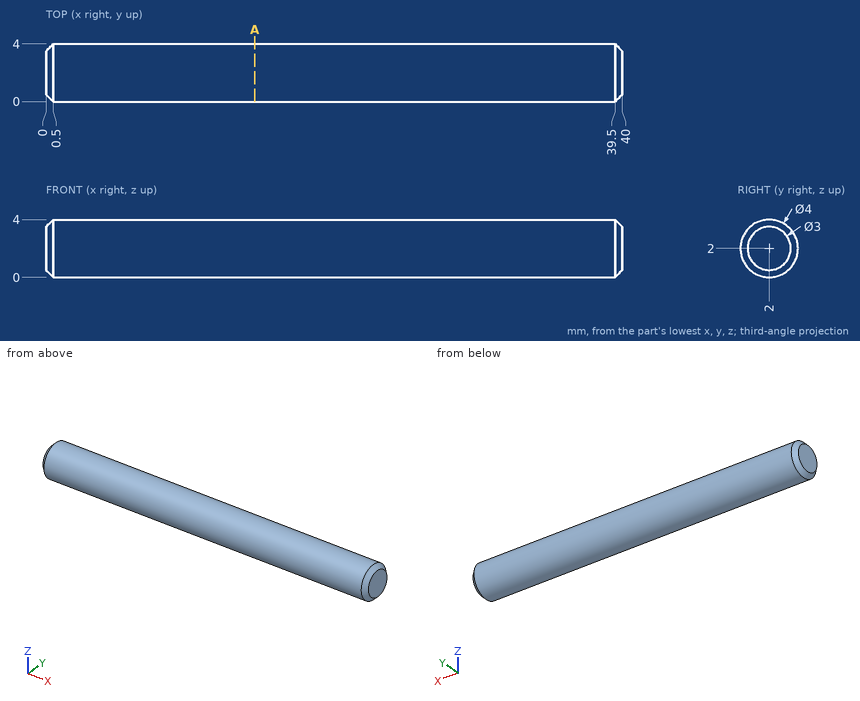
For this review, use the dimensioned drawing (mm, ordinates from the lowest corner) and the shaded views. Coordinates: 2 decimals unless noted, no trailing zeros. Write each loop counter-clockwise with the first axis right and the second up, starting at its lowest first coordinate (ties: lowest second). Pieces come first, ordered by that corner, then holes. Notation, with made-up numbers: (73, -22) - (80, -22) arc R16 cw to (80, 8) - close; hole circle Ø9 at (-22.5, 76.25). An arc over 180 degrees is marked (long way). Answer in a Markdown table with one row per item. Add a question column.
Q1. Consider section A-A on x = 14.5. Give the boundary of the cut face in (y, z).
Q2. Clearance check with a flat-ended pin moving along its axis: pin 1 (1.5 mm diameter, centred on x = 12, z = 3, fed in from -Y). State where the tip first meets the part, or that it passes through.
Q3. To check wall thickness, follow line 1 along Z through (x, y) = (36.5, 1.9); line 2 along Y through (x, z) = (38.5, 3.2); line 3 along Y through (x, z) = (3.5, 2.65). State the ranges of each line that lie inside material, in increasing order. Write a range as from..to.
Answers below:
| question | item | result |
|---|---|---|
| 1 | outline | circle Ø4 at (2, 2) |
| 2 | pin 1 | y = 0.02 |
| 3 | line 1 | 0..4 |
| 3 | line 2 | 0.4..3.6 |
| 3 | line 3 | 0.11..3.89 |
